from build123d import *

# Parameters (mm, degrees)
BOSS_EXTRUDE1_DEPTH                = 20
SKETCH2_W                          = 1.25
SKETCH2_H                          = 6
TAP_DRILL_FOR_M2_5X0_45_TAP1_D     = 2.05
TAP_DRILL_FOR_M2_5X0_45_TAP1_DEPTH = 19
CHAMFER1_SIZE                      = 0.5


with BuildPart() as part:
    # Sketch1 → Boss-Extrude1 (new body)
    with BuildSketch(Plane(origin=(0, 20, 0), x_dir=(1, 0, 0), z_dir=(0, 1, 0))):
        Polygon((1.356773133, -2.35), (2.713546265, 0), (1.356773133, 2.35), (-1.356773133, 2.35), (-2.713546265, 0), (-1.356773133, -2.35), align=None)
    extrude(amount=-BOSS_EXTRUDE1_DEPTH)

    # Sketch2 → Revolve1 (revolve)
    with BuildSketch(Plane(origin=(0, 0, 0), x_dir=(-1, 0, 0), z_dir=(0, 0, -1)), mode=Mode.PRIVATE) as revolve1_sk:
        with Locations((-0.625, -3)):
            Rectangle(SKETCH2_W, SKETCH2_H)
    revolve(revolve1_sk.sketch.rotate(Axis((0, -6, 0), (0, 1, 0)), 270), axis=Axis((0, -6, 0), (0, 1, 0)))

    # Tap Drill for M2.5x0.45 Tap1
    with Locations(Plane(origin=(0, 20, 0), x_dir=(1, 0, 0), z_dir=(0, 1, 0))):
        with Locations((0, 0)):
            Hole(TAP_DRILL_FOR_M2_5X0_45_TAP1_D / 2, depth=TAP_DRILL_FOR_M2_5X0_45_TAP1_DEPTH)

    # Chamfer1
    chamfer1_edges = [part.edges().sort_by_distance(p)[0] for p in [
        (0, -6, -1.25),
        (1.025, 20, 0),
    ]]
    chamfer(chamfer1_edges, length=CHAMFER1_SIZE)


solid = part.part
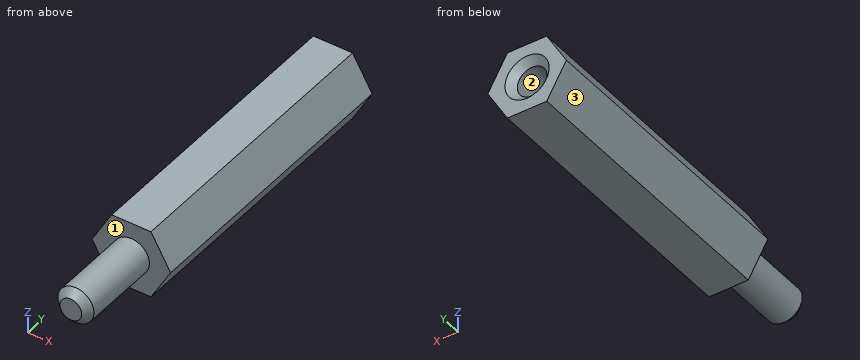
Geometry check sheet. Reference: the model listing, model coordinates, mm. Face numbers are marked on the shaded views. A direction names the side the tool comes from. Give positions to 0.01 mm unless a question says otherwise; leave off trailing zeros. Loops run counter-clockwise (first coordinate to the right, second up) from the corner with the lowest first, then second, coordinate; pieces in that order, holes last. Notation, with made-up numbers: M -9,-24.75 L 16,-24.75 A14 ccw 16,1.25 Z; hole C 29.5,4.25 d3. An arc over 180 degrees is marked long. Answer as a JSON object with one key per item and string values. Group by question number.
Item 1: Sectioned sample at D-D on z = -1.9. Record the boundary of the cut face in (x, y), plus the area to 3 significant figures.
Item 2: Sectioned sample at B-B on x = 0. Record the boundary of the cut face in (y, z) (3 decimals).
Item 3: Access from +Z, -Z, +X, -X, +Y, -Y to the whole of each face (thin tool, end or side, straight path). Record for the marked faces 1, 2 and 3.
Item 4: Sectioned sample at A-A on y = 5.5. Record the boundary of the cut face in (x, z) (3 decimals).
Item 5: Sectioned sample at C-C on y = -1.5. Record the boundary of the cut face in (x, z), plus the area to 3 significant figures.
Item 6: Material ranges on L1, parallel to Z at x = 0, y = 18.5 (3 decimals); L2, parallel to X at y = 1.5, z = 2.05; L3, parallel to Y at x = 0.9, z = -1.8, recorded low to high.
Item 7: Gauge pin test, flat end, axial feed: pin 1 (1 mm diameter, centred on y = 15.5, z = 1.5, fed in from +X). Record the tip position at first contact, or that the pin passes through.
Findings below:
{
 "1": {"outline": "M -1.62,0 L 1.62,0 L 1.62,20 L -1.62,20 Z", "area": "64.7 mm2"},
 "2": {"outline": "M -6,-0.75 L -5.5,-1.25 L 0,-1.25 L 0,-2.35 L 20,-2.35 L 20,-1.525 L 19.5,-1.025 L 1,-1.025 L 1,1.025 L 19.5,1.025 L 20,1.525 L 20,2.35 L 0,2.35 L 0,1.25 L -5.5,1.25 L -6,0.75 Z"},
 "3": {"face 1": "-Y", "face 2": "+Y", "face 3": "-Z, -X, +Y, -Y"},
 "4": {"outline": "M -2.714,0 L -1.357,-2.35 L 1.357,-2.35 L 2.714,0 L 1.357,2.35 L -1.357,2.35 Z; hole C 0,0 d2.05"},
 "5": {"outline": "C 0,0 d2.5", "area": "4.91 mm2"},
 "6": {"L1": "-2.35 to -1.025, 1.025 to 2.35", "L2": "-1.53 to 1.53", "L3": "0 to 20"},
 "7": {"pin 1": "x = 2.14"}
}
